Source: CAD feature listing. Evaluate the final solid. Frame: model axes, mm. A direction names the side the tool comes from. Give positions to 0.01 mm unless a question says otherwise; leave off trailing zeros. Order: outer loops, then holes, each group sorted by start corner. A loop starts at its lowest first (then second) coordinate and runs counter-clockwise, first axis right, second up. Notation, with made-up numbers: M 33,69 L 78,69 A6 ccw 78,79 Z; hole C 26,8 d3. An arc over 180 degrees is marked long. Answer as a JSON object with one key per item and string values. Group by question number.
1. Section query A-A (x = -120.65). Output: boundary loops of the cut face in (y, z).
2. Set-up query: faces 1 (the flat face through (-95, 3, -76.2)), 2 (the cylindrical face through (-109.755, 3.131, -25.968)). Return all of +Z, -Z, +X, -X, +Y, -Y with unobstructed straight access to the full face (end or side cutting, diameter ignored); none if empty.
3. Pull-direction query (X, two-part tool) for faces 3 (the cylindrical face through (-106.734, 3.131, -32.865)), 4 (the flat face through (-127, 3, -26.037)), 5 (the flat face through (-76.2, 3, -102)); classes: +X half, -X half, draft (parallel to the pull), parting line (faces both ways), or undercut.
4. Section query C-C (x = -31.75). Count the separate pieces of the cut face and the enclosed holes in it, plus the area to 3 significant figures.
5. Section query B-B (z = -88.9). Output: boundary loops of the cut face in (x, y).
6. Pin query (flat end, axial travel): P1, Ø3, axis at x = -127, y = 3, coming from the -Z side; P2, Ø11, axis at x = -12.7, z = -127, coming from the -Y side; P3, Ø2, axis at x = -113, y = 5.5, coming from the -Z side; P4, Ø3, axis at y = 2, z = -29, coming from the -X side. Return the tip coordinate at first contact, or that it passes through.
7. Material intervals for L1, parallel to Z at x = -120.65, y = 3.75; L2, parallel to Z at x = -127, y = 2; L3, parallel to X at y = 3.75, z = -123, sorted ascending. Write a range as [from, to].
Autodesk Inventor part; units mm, degrees
ref_plane "YZ Plane" through (0, 0, 0) normal (1, 0, 0) x (0, 1, 0)
ref_plane "XZ Plane" through (0, 0, 0) normal (0, 1, 0) x (-1, 0, 0)
ref_plane "XY Plane" through (0, 0, 0) normal (0, 0, 1) x (1, 0, 0)
sketch "Sketch1" plane through (0, 0, 0) normal (0, 1, 0) x (-1, 0, 0)
  line L0 (0, 0) -> (139.7, 0)
  line L1 (139.7, 0) -> (139.7, -152.4)
  line L2 (139.7, -152.4) -> (0, -152.4)
  line L3 (0, -152.4) -> (0, 0)
  line L4 (139.7, -152.4) -> (127, -152.4)
  line L5 (114.3, -76.2) -> (114.3, -26.0366)
  line L6 (114.3, -26.0366) -> (139.7, -26.0366)
  line L7 (139.7, -26.0366) -> (139.7, -152.4)
  line L8 (127, -152.4) -> (76.2, -152.4)
  line L9 (76.2, -127) -> (76.2, -76.2)
  line L10 (76.2, -76.2) -> (114.3, -76.2)
  line L11 (76.2, -152.4) -> (50.8, -152.4)
  line L12 (50.8, -152.4) -> (50.8, -127)
  line L13 (50.8, -127) -> (76.2, -127)
  circle A0 centre (12.7, -12.7) radius 6.35 construction
  circle A1 centre (12.7, -31.75) radius 6.35 construction
  circle A2 centre (12.7, -50.8) radius 6.35 construction
  circle A3 centre (12.7, -69.85) radius 6.35 construction
  circle A4 centre (12.7, -88.9) radius 6.35 construction
  circle A5 centre (12.7, -107.95) radius 6.35 construction
  circle A6 centre (12.7, -127) radius 6.35 construction
  circle A7 centre (31.75, -12.7) radius 6.35 construction
  circle A8 centre (31.75, -31.75) radius 6.35 construction
  circle A9 centre (31.75, -50.8) radius 6.35 construction
  circle A10 centre (31.75, -69.85) radius 6.35 construction
  circle A11 centre (31.75, -88.9) radius 6.35 construction
  circle A12 centre (31.75, -107.95) radius 6.35 construction
  circle A13 centre (31.75, -127) radius 6.35 construction
  circle A14 centre (12.7, -12.7) radius 6.873
  circle A15 centre (12.7, -31.75) radius 6.8857
  circle A16 centre (12.7, -50.8) radius 6.8984
  circle A17 centre (12.7, -69.85) radius 6.9111
  circle A18 centre (12.7, -88.9) radius 6.9238
  circle A19 centre (12.7, -107.95) radius 6.9365
  circle A20 centre (12.7, -127) radius 6.9492
  circle A21 centre (31.75, -12.7) radius 6.9619
  circle A22 centre (31.75, -31.75) radius 6.9746
  circle A23 centre (31.75, -50.8) radius 6.9873
  circle A24 centre (31.75, -69.85) radius 7
  circle A25 centre (31.75, -88.9) radius 7.0127
  circle A26 centre (31.75, -107.95) radius 7.0254
  circle A27 centre (31.75, -127) radius 7.0381
  circle A28 centre (50.8, -12.7) radius 7.0635
  circle A29 centre (50.8, -31.75) radius 7.0635
  circle A30 centre (50.8, -50.8) radius 7.0762
  circle A31 centre (50.8, -69.85) radius 7.0889
  circle A32 centre (50.8, -88.9) radius 7.1016
  circle A33 centre (50.8, -107.95) radius 7.0045
  circle A34 centre (76.2, -12.7) radius 6.35
  circle A35 centre (76.2, -31.75) radius 6.35
  circle A36 centre (76.2, -50.8) radius 6.35
  line L14 (6.4177, -6.5588) -> (6.4177, -14.6901) construction
  line L15 (8.0052, -4.9713) -> (8.0052, -13.1026) construction
  circle A37 centre (133.35, -6.35) radius 1.778
  circle A38 centre (133.35, -12.7) radius 1.7907
  circle A39 centre (133.35, -19.05) radius 1.8034
  circle A40 centre (127, -6.35) radius 1.8161
  circle A41 centre (127, -12.7) radius 1.8288
  circle A42 centre (127, -19.05) radius 1.8415
  circle A43 centre (120.65, -6.35) radius 1.8542
  circle A44 centre (120.65, -12.7) radius 1.8669
  circle A45 centre (120.65, -19.05) radius 1.8796
  circle A46 centre (114.3, -6.35) radius 1.8923
  circle A47 centre (114.3, -12.7) radius 1.8669
  circle A48 centre (114.3, -19.05) radius 1.8796
  circle A49 centre (107.95, -6.35) radius 1.8923
  circle A50 centre (107.95, -12.7) radius 1.8669
  circle A51 centre (107.95, -19.05) radius 1.8796
  circle A52 centre (107.95, -25.4) radius 1.8923
  circle A53 centre (107.95, -31.75) radius 1.65
  circle A54 centre (107.95, -38.1) radius 1.7
  circle A55 centre (107.95, -44.45) radius 1.75
  circle A56 centre (107.95, -50.8) radius 2.15
  circle A57 centre (107.95, -57.15) radius 2.2
  circle A58 centre (107.95, -63.5) radius 2.25
  dimension "d0" = 139.7
  dimension "d1" = 152.4
  dimension "d3" = 127
  dimension "d5" = 76.2
  dimension "d7" = 25.4
  dimension "d8" = 12.7
  dimension "d9" = 12.7
  dimension "d10" = 12.7
  dimension "d13" = 19.05
  dimension "d16" = 19.05
  dimension "d19" = 13.746
  dimension "d20" = 13.7714
  dimension "d21" = 13.7968
  dimension "d22" = 13.8222
  dimension "d23" = 13.8476
  dimension "d24" = 13.873
  dimension "d25" = 13.8984
  dimension "d26" = 13.9238
  dimension "d27" = 13.9492
  dimension "d28" = 13.9746
  dimension "d29" = 14
  dimension "d30" = 14.0254
  dimension "d31" = 14.0508
  dimension "d32" = 14.0762
  dimension "d33" = 14.127
  dimension "d34" = 14.127
  dimension "d35" = 14.1524
  dimension "d36" = 14.1778
  dimension "d37" = 14.2032
  dimension "d38" = 14.009
  dimension "d39" = 12.7
  dimension "d40" = 12.7
  dimension "d41" = 12.7
  dimension "d44" = 50.8
  dimension "d45" = 25.4
  dimension "d46" = 25.4
  dimension "d47" = 3.556
  dimension "d48" = 6.35
  dimension "d49" = 6.35
  dimension "d50" = 3.5814
  dimension "d51" = 6.35
  dimension "d52" = 3.6068
  dimension "d53" = 6.35
  dimension "d54" = 3.6322
  dimension "d55" = 6.35
  dimension "d56" = 3.6576
  dimension "d57" = 3.683
  dimension "d58" = 3.7084
  dimension "d59" = 6.35
  dimension "d60" = 3.7338
  dimension "d61" = 3.7592
  dimension "d62" = 3.7846
  dimension "d63" = 6.35
  dimension "d64" = 3.7338
  dimension "d65" = 3.7592
  dimension "d66" = 3.7846
  dimension "d67" = 6.35
  dimension "d68" = 3.7338
  dimension "d69" = 3.7592
  dimension "d70" = 3.7846
  dimension "d71" = 6.35
  dimension "d72" = 3.3
  dimension "d73" = 3.4
  dimension "d74" = 3.5
extrude "Extrusion1" add sketch "Sketch1" along normal blind 6.35 contours L0 L1 L6 L5 L10 L9 L13 L12 L2 L3
sketch "Sketch2" plane through (0, 6.35, 0) normal (0, 1, 0) x (1, 0, 0)
  line L0 (-4.5975, 9.3875) -> (-4.5975, 17.5188) construction
  line L1 (-4.5975, 17.5188) -> (-1.4235, 17.5188) construction
  line L2 (-1.4235, 17.5188) -> (-1.4235, 9.3875) construction
  line L3 (-1.4235, 9.3875) -> (-4.5975, 9.3875) construction
  point P0 (0, 0)
sketch "Sketch3" plane through (0, 6.35, 0) normal (0, 1, 0) x (1, 0, 0)
  point P0 (0, 0)
sketch "Sketch4" plane through (0, 6.35, 0) normal (0, 1, 0) x (1, 0, 0)
  line L0 (-95.25, 12.7) -> (-95.2246, 12.7)
  line L1 (-95.2246, 12.7) -> (-95.2246, 38.1)
  line L2 (-95.2246, 38.1) -> (-95.25, 38.1)
  line L3 (-95.25, 38.1) -> (-95.25, 12.7)
  line L4 (-139.7, 26.0366) -> (-139.7, 0)
  line L5 (-139.7, 0) -> (0, 0)
  dimension "d84" = 0.0254
  dimension "d85" = 25.4
  dimension "d86" = 44.45
  dimension "d87" = 12.7
extrude "Extrusion2" cut sketch "Sketch4" against normal through all
properties part number "Test laser cutter tolerances"
Answer sheet:
{
 "1": {"outline": "M 0,-26.04 L 6.35,-26.04 L 6.35,-20.93 L 0,-20.93 Z; M 0,-17.17 L 6.35,-17.17 L 6.35,-14.57 L 0,-14.57 Z; M 0,-10.83 L 6.35,-10.83 L 6.35,-8.2 L 0,-8.2 Z; M 0,-4.5 L 6.35,-4.5 L 6.35,0 L 0,0 Z"},
 "2": {"face 1": "-Z, -X, +Y, -Y", "face 2": "+Y, -Y"},
 "3": {"face 3": "undercut", "face 4": "draft", "face 5": "-X half"},
 "4": {"separate pieces": "8", "enclosed holes": "0", "area": "345 mm^2"},
 "5": {"outline": "M -76.2,0 L -57.9,0 L -57.9,6.35 L -76.2,6.35 Z; M -43.7,0 L -38.76,0 L -38.76,6.35 L -43.7,6.35 Z; M -24.74,0 L -19.62,0 L -19.62,6.35 L -24.74,6.35 Z; M -5.78,0 L 0,0 L 0,6.35 L -5.78,6.35 Z"},
 "6": {"P1": "z = -26.04", "P2": "through", "P3": "z = -76.2", "P4": "x = -114.3"},
 "7": {"L1": "[-26.04, -20.93], [-17.17, -14.57], [-10.83, -8.2], [-4.5, 0]", "L2": "[-26.04, -20.89], [-17.21, -14.53], [-10.87, -8.17], [-4.53, 0]", "L3": "[-76.2, -37.54], [-25.96, -18.38], [-7.02, 0]"}
}
